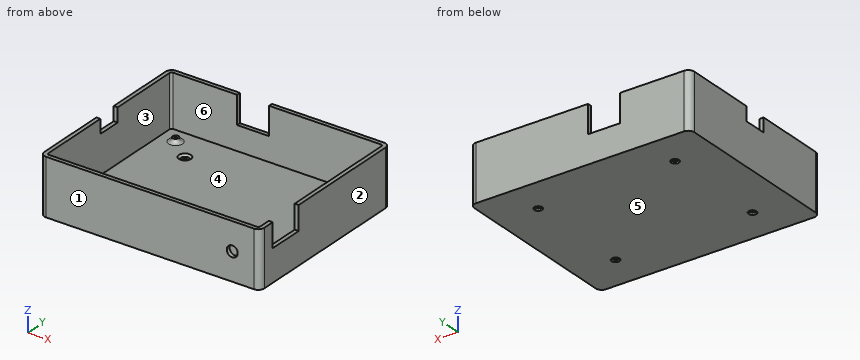
from build123d import *

# Parameters (mm, degrees)
BOSS_EXTRUDE1_DEPTH = 2
BOSS_EXTRUDE2_DEPTH = 26
SKETCH5_R           = 1.5
SKETCH5_R_2         = 0.5
BOSS_EXTRUDE4_DEPTH = 4
FILLET2_R           = 2
SKETCH9_W           = 16
SKETCH9_H           = 14
CUT_EXTRUDE3_DEPTH  = 2.5
SKETCH11_R          = 2.75
CUT_EXTRUDE5_DEPTH  = 2.5
CUT_EXTRUDE6_REACH  = 124.102
SKETCH12_W          = 7
SKETCH12_H          = 12
SKETCH13_W          = 12
SKETCH13_H          = 18
CUT_EXTRUDE7_DEPTH  = 10
SKETCH14_R          = 2
CUT_EXTRUDE8_DEPTH  = 10
CHAMFER1_SIZE       = 1


with BuildPart() as part:
    # Sketch2 → Boss-Extrude1 (new body)
    with BuildSketch(Plane.XY):
        with BuildLine():
            Line((-52, -45), (52, -45))
            ThreePointArc((52, -45), (54.121320344, -44.121320344), (55, -42))
            Line((55, -42), (55, 42))
            ThreePointArc((55, 42), (54.121320344, 44.121320344), (52, 45))
            Line((52, 45), (-52, 45))
            ThreePointArc((-52, 45), (-54.121320344, 44.121320344), (-55, 42))
            Line((-55, 42), (-55, -42))
            ThreePointArc((-55, -42), (-54.121320344, -44.121320344), (-52, -45))
        make_face()
    extrude(amount=BOSS_EXTRUDE1_DEPTH)

    # Sketch3 → Boss-Extrude2 (add)
    with BuildSketch(Plane.XY.offset(2)):
        with BuildLine():
            Line((55, -42), (55, 42))
            ThreePointArc((55, 42), (54.121320344, 44.121320344), (52, 45))
            Line((52, 45), (-52, 45))
            ThreePointArc((-52, 45), (-54.121320344, 44.121320344), (-55, 42))
            Line((-55, 42), (-55, -42))
            ThreePointArc((-55, -42), (-54.121320344, -44.121320344), (-52, -45))
            Line((-52, -45), (52, -45))
            ThreePointArc((52, -45), (54.121320344, -44.121320344), (55, -42))
        make_face()
        with BuildLine():
            Line((52, 43), (-52, 43))
            ThreePointArc((-52, 43), (-52.707106781, 42.707106781), (-53, 42))
            Line((-53, 42), (-53, -42))
            ThreePointArc((-53, -42), (-52.707106781, -42.707106781), (-52, -43))
            Line((-52, -43), (52, -43))
            ThreePointArc((52, -43), (52.707106781, -42.707106781), (53, -42))
            Line((53, -42), (53, 42))
            ThreePointArc((53, 42), (52.707106781, 42.707106781), (52, 43))
        make_face(mode=Mode.SUBTRACT)
    extrude(amount=BOSS_EXTRUDE2_DEPTH)

    # Sketch5 → Boss-Extrude4 (add)
    # profile 1 of 4: a face of its own
    with BuildSketch(Plane(origin=(0, 0, 0), x_dir=(-1, 0, 0), z_dir=(0, 0, -1))):
        with Locations((45, 35)):
            Circle(SKETCH5_R)
        with Locations((45, 35)):
            Circle(SKETCH5_R_2, mode=Mode.SUBTRACT)
    # profile 2 of 4: a face of its own
    with BuildSketch(Plane(origin=(0, 0, 0), x_dir=(-1, 0, 0), z_dir=(0, 0, -1))):
        with Locations((-45, 35)):
            Circle(SKETCH5_R)
        with Locations((-45, 35)):
            Circle(SKETCH5_R_2, mode=Mode.SUBTRACT)
    # profile 3 of 4: a face of its own
    with BuildSketch(Plane(origin=(0, 0, 0), x_dir=(-1, 0, 0), z_dir=(0, 0, -1))):
        with Locations((-45, -35)):
            Circle(SKETCH5_R)
        with Locations((-45, -35)):
            Circle(SKETCH5_R_2, mode=Mode.SUBTRACT)
    # profile 4 of 4: a face of its own
    with BuildSketch(Plane(origin=(0, 0, 0), x_dir=(-1, 0, 0), z_dir=(0, 0, -1))):
        with Locations((45, -35)):
            Circle(SKETCH5_R)
        with Locations((45, -35)):
            Circle(SKETCH5_R_2, mode=Mode.SUBTRACT)
    extrude(amount=-BOSS_EXTRUDE4_DEPTH)

    # Fillet2
    fillet2_edges = [part.edges().sort_by_distance(p)[0] for p in [
        (46.5, 35, 2),
        (46.5, -35, 2),
        (-43.5, -35, 2),
        (-43.5, 35, 2),
    ]]
    fillet(fillet2_edges, radius=FILLET2_R - 0.0001)  # a hair under: the kernel refuses the full size

    # Sketch9 → Cut-Extrude3 (cut)
    with BuildSketch(Plane(origin=(0, 43, 0), x_dir=(-1, 0, 0), z_dir=(0, -1, 0))):
        with Locations((12, -21)):
            Rectangle(SKETCH9_W, SKETCH9_H)
    extrude(amount=-CUT_EXTRUDE3_DEPTH, mode=Mode.SUBTRACT)

    # Sketch11 → Cut-Extrude5 (cut)
    with BuildSketch(Plane(origin=(0, -45, 0), x_dir=(-1, 0, 0), z_dir=(0, -1, 0))):
        with Locations(Location((-41.126488164, -14, 0), (0, 0, 90))):
            Circle(SKETCH11_R)
    extrude(amount=-CUT_EXTRUDE5_DEPTH, mode=Mode.SUBTRACT)

    # Sketch12 → Cut-Extrude6 (cut, up to next)
    with BuildSketch(Plane.ZY.offset(55), mode=Mode.PRIVATE) as cut_extrude6_sk1:
        with Locations((24.5, 0)):
            Rectangle(SKETCH12_W, SKETCH12_H)
    cut_extrude6_tool1 = extrude(cut_extrude6_sk1.sketch, amount=-CUT_EXTRUDE6_REACH, mode=Mode.PRIVATE) & part.part
    add(cut_extrude6_tool1.solids().sort_by_distance((-55, 0, 24.5))[0], mode=Mode.SUBTRACT)

    # Sketch13 → Cut-Extrude7 (cut)
    with BuildSketch(Plane(origin=(55, 0, 0), x_dir=(0, 0, -1), z_dir=(1, 0, 0))):
        with Locations((-22, -27.190217321)):
            Rectangle(SKETCH13_W, SKETCH13_H)
    extrude(amount=-CUT_EXTRUDE7_DEPTH, mode=Mode.SUBTRACT)

    # Sketch14 → Cut-Extrude8 (cut)
    with BuildSketch(Plane.XY.offset(2)):
        with Locations((-34.243884653, -27.074376311)):
            Circle(SKETCH14_R)
        with Locations((34.243884653, 26.574376311)):
            Circle(SKETCH14_R)
        with Locations((34.243884653, -27.074376311)):
            Circle(SKETCH14_R)
        with Locations((-34.243884653, 26.574376311)):
            Circle(SKETCH14_R)
    extrude(amount=-CUT_EXTRUDE8_DEPTH, mode=Mode.SUBTRACT)

    # Chamfer1
    chamfer1_edges = [part.edges().sort_by_distance(p)[0] for p in [
        (-36.243884653, 26.574376311, 2),
        (32.243884653, -27.074376311, 2),
        (32.243884653, 26.574376311, 2),
        (-36.243884653, -27.074376311, 2),
    ]]
    chamfer(chamfer1_edges, length=CHAMFER1_SIZE)


solid = part.part
Design review of the part built by this model. Coordinates are the model's own, in mm. Face numbers are marked on the shaded views. A direction names the side the tool comes from. Give positions to 0.01 mm unless a question says otherwise; leave off trailing zeros. Write each loop counter-clockwise with the first axis right and the second up, starting at its lowest first coordinate (ties: lowest second). Pieces come first, ordered by that corner, then holes. Notation, with made-up numbers: M 71,53 L 118,53 A31 cw 118,80 Z; hole C 13.25,8.5 d4. An arc over 180 degrees is marked long. Return JSON: item names as keys, results as strings. Group by question number.
Item 1: Take a section at A-A (x = -10.5). Give the boundary of the cut face in (y, z), plus the area to 3 significant figures.
Item 2: Clearance check with flat-ended pins moving along their axes: pin 1 Ø0.9 at (x, y) = (44.5, -34.5) entering from +Z; pin 2 Ø0.6 at (x, z) = (54, 21.5) entering from +Y; pin 3 Ø0.8 at (x, y) = (45, -35) entering from +Z. State where each tip first meets the part, or that it passes through.
Item 3: Tool access review of the marked faces 5 and 6: name each direction out of +Z, -Z, +X, -X, +Y, -Y from which nothing blocks a thin tool from reaching the whole face with its end or side.
Item 4: Wall thickness on line 1 along X through (y, z) = (-26, 9.5); line 2 along Y through (x, z) = (-41, 10.5); line 3 along Y through (x, z) = (45, 2.7): over which ranges is each line inside the solid? List them lowest first.
Item 5: Take a section at C-C (y = 16.5). Give the boundary of the cut face in (x, z).
Item 6: Take a section at B-B (z = 5.5). Give the boundary of the cut face in (x, y), plus the area to 3 significant figures.
Item 7: The part is to be moulded in two halves that separate along X. For the marked faces 1, 2, 3 and 4, say which applies: pulls with the +X half, pulls with the -X half, needs draft (parallel to the pull), parting line crosses it, or undercut.
Return value:
{
 "1": {"outline": "M -45,0 L 45,0 L 45,14 L 43,14 L 43,2 L -43,2 L -43,28 L -45,28 Z", "area": "256 mm2"},
 "2": {"pin 1": "stops at z = 4", "pin 2": "stops at y = 44.47", "pin 3": "stops at z = 2"},
 "3": {"face 5": "-Z, +X, -X, +Y, -Y", "face 6": "+Z"},
 "4": {"line 1": "x = -55 to -53, 53 to 55", "line 2": "y = -45 to -43, 43 to 45", "line 3": "y = -45 to -43, -36.98 to -35.5, -34.5 to -33.02, 33.02 to 34.5, 35.5 to 36.98, 43 to 45"},
 "5": {"outline": "M -55,0 L 55,0 L 55,28 L 53,28 L 53,2 L -53,2 L -53,28 L -55,28 Z"},
 "6": {"outline": "M -55,-42 A3 ccw -52,-45 L 52,-45 A3 ccw 55,-42 L 55,42 A3 ccw 52,45 L -52,45 A3 ccw -55,42 Z; hole M -53,-42 A1 ccw -52,-43 L 52,-43 A1 ccw 53,-42 L 53,42 A1 ccw 52,43 L -52,43 A1 ccw -53,42 Z", "area": "777 mm2"},
 "7": {"face 1": "needs draft", "face 2": "pulls with the +X half", "face 3": "undercut", "face 4": "undercut"}
}
